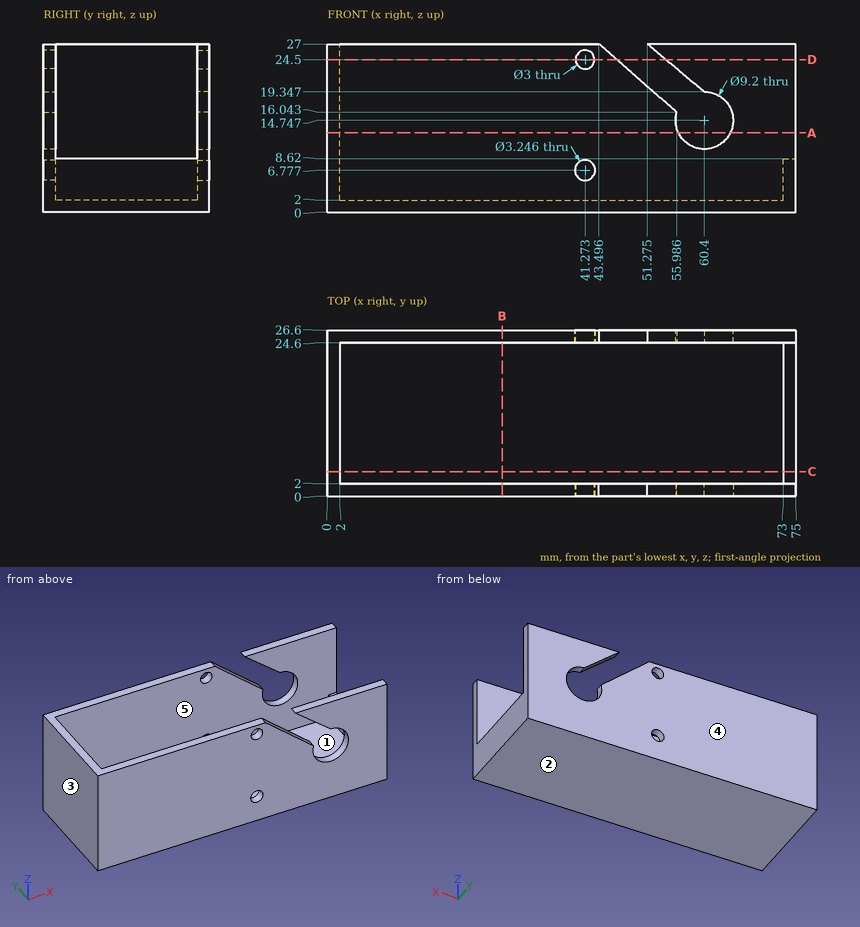
Drawing for the job (mm, zero at the part's lowest x, y, z). A direction names the side the tool comes from. Give positions to 0.01 mm unless a question says otherwise; leave off trailing zeros. Loops run counter-clockwise (first coordinate to the right, second up) from the corner with the lowest first, then second, coordinate; pieces in that order, holes last.
1) Drop flat-ended pins along their axis: P1, Ø1, axis at x = 74, y = 12, coming from the +Z side; P2, Ø2, axis at x = 37, y = 5, coming from the +Z side; P3, Ø3, axis at y = 9, z = 23.5, coming from the +X side. Give the stop position or say it passes through.
Values follow:
P1: stops at z = 8.62
P2: stops at z = 2
P3: stops at x = 2
2) Band-saw the part on B-B on x = 28. List the corners of the cut face in (y, z).
Values follow:
outline: (0, 0) - (26.6, 0) - (26.6, 27) - (24.6, 27) - (24.6, 2) - (2, 2) - (2, 27) - (0, 27) - close
3) Band-saw the part on A-A on z = 12.75. List the corners of the cut face in (x, y), then the cut area to 3 significant figures.
Values follow:
outline: (0, 0) - (56.26, 0) - (56.26, 2) - (2, 2) - (2, 24.6) - (56.26, 24.6) - (56.26, 26.6) - (0, 26.6) - close; (64.54, 0) - (75, 0) - (75, 2) - (64.54, 2) - close; (64.54, 24.6) - (75, 24.6) - (75, 26.6) - (64.54, 26.6) - close
area: 312 mm2
4) Band-saw the part on D-D on z = 24.5. List the corners of the cut face in (x, y) (1 decimal).
Values follow:
outline: (0, 0) - (39.8, 0) - (39.8, 2) - (2, 2) - (2, 24.6) - (39.8, 24.6) - (39.8, 26.6) - (0, 26.6) - close; (42.8, 0) - (46.3, 0) - (46.3, 2) - (42.8, 2) - close; (42.8, 24.6) - (46.3, 24.6) - (46.3, 26.6) - (42.8, 26.6) - close; (54.3, 0) - (75, 0) - (75, 2) - (54.3, 2) - close; (54.3, 24.6) - (75, 24.6) - (75, 26.6) - (54.3, 26.6) - close
5) Two-plate mould, pull along X, no slides. Class the marked faces 3, 4 and 5: released by +X, released by -X, zero draft, split by the parting line, or undercut.
Values follow:
face 3: released by -X
face 4: zero draft
face 5: undercut
6) Band-saw the part on C-C on y = 4. List the corners of the cut face in (x, z).
Values follow:
outline: (0, 0) - (75, 0) - (75, 8.62) - (73, 8.62) - (73, 2) - (2, 2) - (2, 27) - (0, 27) - close
7) 3-axis set-ups, long thin cutter, end or side, ignore diameter. For the marked faces 1 and 2: which of +Z, -Z, +X, -X, +Y, -Y reach the whole face in a straight line?
Values follow:
face 1: +Z
face 2: -Z, +X, -X, +Y, -Y
8) Probe line 1 along Y through (x, z) = (22, 6.75); line 2 along Z through (x, y) = (60.4, 25.1) (1 decimal); line 3 along Z through (x, y) = (52, 5.5). List the from-to ranges inside material, lowest first.
Values follow:
line 1: y = 0 to 2, 24.6 to 26.6
line 2: z = 0 to 10.1, 19.3 to 27
line 3: z = 0 to 2
